Input: part model. Units: mm. Frame: model coordinates. A direction names the side the tool comes from. Round coordinates to 2 decimals unless told otherwise and drop trailing zeros. Order: outer loops, then holes, each group sorted by start corner. A loop starts at its lowest first (then second) coordinate and runs counter-clockwise, first axis right, second up. Notation, with made-up numbers: (29, 18) -> (48, 18) arc R23 cw to (48, 44) -> close; hole circle Ø8 at (22.5, 13.25). An arc over 180 degrees is marked (long way). Use a Markdown table: item, result.
from build123d import *

# Parameters (mm, degrees)
F1_DEPTH  = 60
F2_R      = 4
F3_R      = 4
F4_R      = 25
F5_DEPTH  = 25
F5_FACE_R = 25
F6_DEPTH  = 25


with BuildPart() as f1:
    # F0 (on Front) → F1 (new body)
    with BuildSketch(Plane.XZ):
        with BuildLine():
            Line((49.595254, 69.832447), (-25.404746, 69.832447))
            ThreePointArc((-25.404746, 69.832447), (-43.082416, 62.510116), (-50.404746, 44.832447))
            Line((-50.404746, 44.832447), (-50.404746, -30.167553))
            Line((-50.404746, -30.167553), (24.595254, -30.167553))
            ThreePointArc((24.595254, -30.167553), (42.272923, -22.845223), (49.595254, -5.167553))
            Line((49.595254, -5.167553), (49.595254, 69.832447))
        make_face()
    extrude(amount=F1_DEPTH)

    # F2
    f2_edges = [f1.edges().sort_by_distance(p)[0] for p in [
        (49.595254, -60, 32.332447),
        (12.095254, -60, 69.832447),
        (-43.082416, -60, 62.510116),
        (-50.404746, -60, 7.332447),
        (-12.904746, -60, -30.167553),
        (42.272923, -60, -22.845223),
    ]]
    fillet(f2_edges, radius=F2_R)

    # F3
    f3_edges = [f1.edges().sort_by_distance(p)[0] for p in [
        (49.595254, 0, 32.332447),
        (12.095254, 0, 69.832447),
        (-43.082416, 0, 62.510116),
        (-50.404746, 0, 7.332447),
        (-12.904746, 0, -30.167553),
        (42.272923, 0, -22.845223),
    ]]
    fillet(f3_edges, radius=F3_R)

    # F4 (on face) → F5 (cut)
    with BuildSketch(Plane.XZ.offset(60)):
        with Locations((0, 22.368037)):
            Circle(F4_R)
    extrude(amount=-F5_DEPTH, mode=Mode.SUBTRACT)

    # F5_face (on face) + F4 (on face) → F6 (cut)
    with BuildSketch(Plane(origin=(0, -35, 22.368037), x_dir=(1, 0, 0), z_dir=(0, -1, 0))):
        Circle(F5_FACE_R)
    with BuildSketch(Plane.XZ.offset(60)):
        with Locations((0, 22.368037)):
            Circle(F4_R)
    extrude(amount=-F6_DEPTH, mode=Mode.SUBTRACT)


solid = f1.part
1) Set-up query: faces 1 (the cylindrical face through (11.54, -35.35, 0.19)), 2 (the cylindrical face through (48.45, -58.8, 32.86)). Return all of +Z, -Z, +X, -X, +Y, -Y with unobstructed straight access to the full face (end or side cutting, diameter ignored); none if empty.
Results found:
| item | result |
|---|---|
| face 1 | -Y |
| face 2 | +Z, -Z, +X, -Y |
2) Cut plane A-A on x = 0. Return loops of the section in (y, z), and give its area (3 significant figures).
Results found:
| item | result |
|---|---|
| outline | (-60, -26.17) arc R4 ccw to (-56, -30.17) -> (-4, -30.17) arc R4 ccw to (0, -26.17) -> (0, 65.83) arc R4 ccw to (-4, 69.83) -> (-56, 69.83) arc R4 ccw to (-60, 65.83) -> (-60, 47.37) -> (-10, 47.37) -> (-10, -2.63) -> (-60, -2.63) -> close |
| area | 3,490 mm² |
3) Cut plane C-C on z = 16. Return loops of the section in (x, y), and give its area (3 significant figures).
Results found:
| item | result |
|---|---|
| outline | (-50.4, -56) arc R4 ccw to (-46.4, -60) -> (-24.18, -60) -> (-24.18, -10) -> (24.18, -10) -> (24.18, -60) -> (45.6, -60) arc R4 ccw to (49.6, -56) -> (49.6, -4) arc R4 ccw to (45.6, 0) -> (-46.4, 0) arc R4 ccw to (-50.4, -4) -> close |
| area | 3,570 mm² |
4) Pin query (flat end, axial travel): pin 1 Ø12 at (x, z) = (2.5, 33.5) entering from -Y; pin 2 Ø5 at (y, z) = (-14.5, -10.5) entering from +X. Return the tip coordinate at first contact, or that it passes through.
Results found:
| item | result |
|---|---|
| pin 1 | stops at y = -10 |
| pin 2 | stops at x = 49.43 |
5) Line query: L1, parallel to Z at x = 0, y = -33.5; L2, parallel to X at y = -15, z = 22; L3, parallel to Y at x = -8, z = 11. Output: solid intervals per line, ascending. Write a range as [from, to].
Results found:
| item | result |
|---|---|
| L1 | z = [-30.17, -2.63], [47.37, 69.83] |
| L2 | x = [-50.4, -25], [25, 49.6] |
| L3 | y = [-10, 0] |
6) Cut plane B-B on y = -45.5. Return loops of the section in (x, z), and give its area (3 significant figures).
Results found:
| item | result |
|---|---|
| outline | (-50.4, -30.17) -> (24.6, -30.17) arc R25 ccw to (49.6, -5.17) -> (49.6, 69.83) -> (-25.4, 69.83) arc R25 ccw to (-50.4, 44.83) -> close; hole circle Ø50 at (0, 22.37) |
| area | 7,770 mm² |
